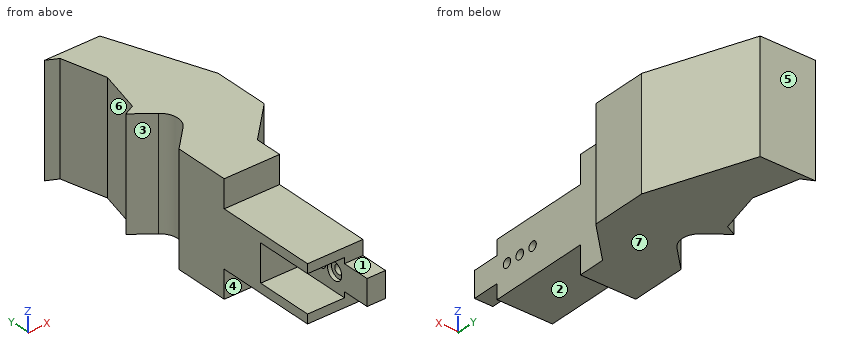
Autodesk Inventor part; units mm, degrees
ref_plane "Work Plane1" through (0, 0, -15) normal (0, 0, 1) x (1, 0, 0)
ref_plane "YZ Plane" through (0, 0, 0) normal (1, 0, 0) x (0, 1, 0)
ref_plane "XZ Plane" through (0, 0, 0) normal (0, 1, 0) x (-1, 0, 0)
sketch "Sketch1" plane through (0, 0, 0) normal (0, 0, 1) x (1, 0, 0)
  line L0 (0, 0) -> (25, 0)
  line L1 (25, 0) -> (25, 40)
  line L2 (25, 40) -> (0, 40)
  line L3 (0, 40) -> (0, 0)
  dimension "d1" = 25
  dimension "d2" = 40
  dimension "d3" = 25
extrude "Extrusion1" add sketch "Sketch1" against normal blind 30
sketch "Sketch2" plane through (25, 0, 0) normal (1, 0, 0) x (0, 0, -1)
  line L0 (0, 0) -> (30, 0)
  circle A0 centre (15, 6.56) radius 2.46
extrude "Extrusion2" cut sketch "Sketch2" against normal blind 30
sketch "Sketch3" plane through (0, 0, 0) normal (-1, 0, 0) x (0, 0, 1)
  line L0 (0, 0) -> (-30, 0)
  line L1 (-25.05, 0) -> (-4.95, 0)
  line L2 (-4.95, 0) -> (-4.95, 33.12)
  line L3 (-4.95, 33.12) -> (-25.05, 33.12)
  line L4 (-25.05, 33.12) -> (-25.05, 0)
  dimension "d11" = 20.1
extrude "Extrusion3" cut sketch "Sketch3" against normal blind 20
sketch "Sketch4" plane through (0, 0, 0) normal (0, -1, 0) x (1, 0, 0)
  line L0 (20, -4.95) -> (20, -25.05)
  line L1 (20, -15) -> (25, -15)
  line L2 (25, 0) -> (25, -30)
  line L3 (20, -8.025) -> (25, -8.025)
  line L4 (25, -8.025) -> (25, -21.975)
  line L5 (25, -21.975) -> (20, -21.975)
  line L6 (20, -21.975) -> (20, -8.025)
  line L7 (20, -8.025) -> (25, -21.975) construction
  line L8 (25, -8.025) -> (20, -21.975) construction
  line L9 (25, -12.54) -> (25, -17.46)
  point P0 (0, 0)
  point P1 (22.5, -15)
  dimension "d14" = 13.95
extrude "Extrusion4" add sketch "Sketch4" along normal blind 15
sketch "Sketch5" plane through (20, 0, 0) normal (-1, 0, 0) x (0, 0, 1)
  circle A0 centre (-15, 6.56) radius 2.46
  circle A1 centre (-15, 6.56) radius 4.7025
  circle A2 centre (-15, 6.56) radius 2.46
  circle A3 centre (-15, 6.56) radius 2.46
  point P0 (0, 0)
  dimension "d17" = 9.405
extrude "Extrusion5" cut sketch "Sketch5" against normal blind 2.1
sketch "Sketch6" plane through (25, 0, 0) normal (1, 0, 0) x (0, 0, -1)
  circle A0 centre (15, 6.56) radius 4.7025
  line L0 (15, 6.56) -> (15, 23.56)
  circle A1 centre (15, 23.56) radius 2.46
  point P0 (0, 0)
  dimension "d20" = 17
  dimension "d21" = 4.92
extrude "Extrusion6" cut sketch "Sketch6" against normal blind 10 contours A1
sketch "Sketch7" plane through (20, 0, 0) normal (-1, 0, 0) x (0, 0, 1)
  circle A0 centre (-15, 23.56) radius 2.46
  circle A1 centre (-15, 23.56) radius 4.7025
  point P0 (0, 0)
  dimension "d24" = 9.405
extrude "Extrusion7" cut sketch "Sketch7" against normal blind 2.1
sketch "Sketch9" plane through (25, 0, 0) normal (1, 0, 0) x (0, 0, -1)
  circle A0 centre (15, 6.56) radius 2.46
  circle A1 centre (15, 6.56) radius 2.46
  circle A2 centre (15, 23.56) radius 2.46
  circle A3 centre (15, 23.56) radius 2.46
  line L0 (30, 40) -> (30, 0)
  line L1 (30, 0) -> (30, 40)
  line L2 (30, 40) -> (0, 40)
  line L3 (0, 40) -> (0, 0)
  line L4 (0, 0) -> (8.025, 0)
  line L5 (21.975, 0) -> (21.975, -15)
  line L6 (21.975, -15) -> (8.025, -15)
  line L7 (8.025, -15) -> (8.025, 0)
  line L8 (0, 0) -> (8.025, 0)
  line L9 (21.975, 0) -> (30, 0)
extrude "Extrusion8" add sketch "Sketch9" along normal blind 5
sketch "Sketch10" plane through (0, 40, 0) normal (0, 1, 0) x (1, 0, 0)
  line L0 (0, 30) -> (30, 30)
  line L1 (30, 0) -> (0, 0)
  line L2 (0, 30) -> (30, 30)
  line L3 (30, 30) -> (30, 0)
  line L4 (30, 0) -> (0, 0)
  line L5 (0, 0) -> (0, 30)
extrude "Extrusion9" add sketch "Sketch10" along normal blind 30
sketch "Sketch12" plane through (30, 0, 0) normal (1, 0, 0) x (0, 0, -1)
  circle A0 centre (15, 6.56) radius 2.46
  line L0 (15, 6.56) -> (15, 15.06)
  circle A1 centre (15, 15.06) radius 2.525
  point P0 (0, 0)
  dimension "d31" = 8.5
  dimension "d33" = 5.05
extrude "Extrusion10" cut sketch "Sketch12" against normal blind 30 contours A1
sketch "Sketch15" plane through (0, 0, -25.05) normal (-1, 0, 0) x (0, 0, 1)
  line L0 (0, 33.12) -> (20.1, 33.12)
  line L1 (20.1, 33.12) -> (20.1, 0)
  line L2 (0, 33.12) -> (20.1, 33.12)
  line L3 (20.1, 33.12) -> (20.1, 31.1)
  line L4 (20.1, 31.1) -> (0, 31.1)
  line L5 (0, 31.1) -> (0, 33.12)
  point P0 (25.05, 0)
  dimension "d57" = 2.02
extrude "Extrusion13" add sketch "Sketch15" against normal blind 20
sketch "Sketch17" plane through (0, 0, 0) normal (0, 0, 1) x (1, 0, 0)
  line L0 (0, 70) -> (30, 70)
  line L1 (30, 70) -> (50.0622, 90.0622)
  line L2 (30, 70) -> (80, 70) construction
  line L3 (11.9522, 97.2454) -> (0, 85.2932)
  line L4 (0, 70) -> (0, 85.2932)
  line L5 (0, 70) -> (0, 0)
  line L6 (0, 70) -> (30, 70)
  line L7 (10.923, 112.2849) -> (0, 120.567)
  line L8 (50.0622, 105.3553) -> (50.0622, 120.567)
  line L9 (50.0622, 105.3553) -> (50.0622, 90.0622)
  arc A0 (11.9522, 97.2454) -> (10.923, 112.2849) centre (4.8811, 104.3165) ccw
  line L10 (0, 174.567) -> (30, 174.567)
  line L11 (30, 174.567) -> (50.0622, 120.567)
  line L12 (6, 171.567) -> (0, 174.567)
  line L13 (6, 123.567) -> (0, 120.567)
  line L14 (6, 123.567) -> (12, 147.567)
  line L15 (6, 171.567) -> (12, 147.567)
  dimension "d61" = 45
  dimension "d62" = 32.0271
  dimension "d72" = 10
extrude "Extrusion14" add sketch "Sketch17" against normal blind 30
sketch "Sketch24" plane through (0, 0, 0) normal (0, 0, 1) x (1, 0, 0)
  line L0 (30, 70) -> (50.0622, 90.0622)
  line L1 (30, 70) -> (50.0622, 90.0622)
  line L2 (50.0622, 90.0622) -> (50.0622, 120.567)
  line L3 (50.0622, 90.0622) -> (50.0622, 120.567)
  line L4 (30, 174.567) -> (50.0622, 120.567)
  line L5 (50.0622, 120.567) -> (30, 174.567)
  line L6 (30, 174.567) -> (0, 174.567)
  line L7 (30, 174.567) -> (0, 174.567)
  line L8 (0, 174.567) -> (6, 171.567)
  line L9 (0, 174.567) -> (6, 171.567)
  line L10 (12, 147.567) -> (6, 171.567)
  line L11 (6, 171.567) -> (12, 147.567)
  line L12 (12, 147.567) -> (6, 123.567)
  line L13 (12, 147.567) -> (6, 123.567)
  line L14 (6, 123.567) -> (0, 120.567)
  line L15 (6, 123.567) -> (0, 120.567)
  line L16 (0, 120.567) -> (10.923, 112.2849)
  line L17 (0, 120.567) -> (10.923, 112.2849)
  line L18 (0, 85.2932) -> (11.9522, 97.2454)
  line L19 (11.9522, 97.2454) -> (0, 85.2932)
  line L20 (0, 85.2932) -> (0, 55.2932)
  line L21 (0, 0) -> (0, 85.2932)
  line L22 (0, 55.2932) -> (30, 55.2932)
  line L23 (30, 0) -> (30, 70)
  line L24 (30, 55.2932) -> (30, 70)
  arc A0 (11.9522, 97.2454) -> (10.923, 112.2849) centre (4.8811, 104.3165) ccw
  dimension "d106" = 30
extrude "Extrusion15" add sketch "Sketch24" along normal blind 15
ref_plane "Work Plane1" through (0, 0, -15) normal (0, 0, 1) x (1, 0, 0)
mirror "Mirror1" about plane through (0, 0, -15) normal (0, 0, 1) of "Extrusion15"
properties part number "rec_c_48mm_x_60mm"
Input: part model. Units: mm. Frame: model coordinates. Face numbers are marked on the shaded views. A direction names the side the tool comes from. Coordinates: 2 decimals unless noted, no trailing zeros. Write each loop counter-clockwise with the first axis right and the second up, starting at its lowest first coordinate (ties: lowest second). Pieces come first, ordered by that corner, then holes. Notation, with made-up numbers: M -40,-6.5 L -29,-6.5 A33 ccw -29,32.5 Z; hole C -2.5,70 d7. An arc over 180 degrees is marked long. Use one line per item in the form item = value.
Q1. Section D-D (x = 9). Return loops of the section in (y, z), plus the area to 3 significant figures.
Answer below:
outline = M 0,-30 L 55.29,-30 L 55.29,-45 L 94.29,-45 L 94.29,15 L 55.29,15 L 55.29,0 L 0,0 L 0,-4.95 L 31.1,-4.95 L 31.1,-25.05 L 0,-25.05 Z; M 113.74,-45 L 135.57,-45 L 135.57,15 L 113.74,15 Z; M 159.57,-45 L 174.57,-45 L 174.57,15 L 159.57,15 Z
area = 5,580 mm²
Q2. Draft query along Y for the marked faces 4, 5, 6 and 7. Return one class per face: released by +Y, released by -Y, zero draft, split by the parting line, or undercut.
Answer below:
face_4 = released by -Y
face_5 = released by +Y
face_6 = undercut
face_7 = zero draft
Q3. Set-up query: the marked faces 1, 2 and 3. Return all of +Z, -Z, +X, -X, +Y, -Y with unobstructed straight access to the full face (end or side cutting, diameter ignored); none if empty.
Answer below:
face_1 = +Z, +X, -X, -Y
face_2 = -Z, +X, -X, -Y
face_3 = +Z, -Z, -X
Q4. Section B-B (x = 24.5). Return loops of the section in (y, z) (3 decimals), plus the area to 3 significant figures.
Answer below:
outline = M -15,-21.975 L 0,-21.975 L 0,-30 L 55.293,-30 L 55.293,-45 L 174.567,-45 L 174.567,15 L 55.293,15 L 55.293,0 L 0,0 L 0,-8.025 L -15,-8.025 Z; hole C 6.56,-15 d4.92; hole C 15.06,-15 d5.05; hole C 23.56,-15 d4.92
area = 8,970 mm²
Q5. Section A-A (y = 23.56). Return loops of the section in (x, z), plus the area to 3 significant figures.
Answer below:
outline = M 0,-30 L 30,-30 L 30,-17.46 L 22.1,-17.46 L 22.1,-19.7 L 20,-19.7 L 20,-25.05 L 0,-25.05 Z; M 0,-4.95 L 20,-4.95 L 20,-10.3 L 22.1,-10.3 L 22.1,-12.54 L 30,-12.54 L 30,0 L 0,0 Z
area = 439 mm²
Q6. Material intervals for probe 1 along Y at (x, z) = (27, -15) (3 decimals); probe 2 along Y at (x, z) = (21.65, -15) (1 decimal); probe 3 along X at (y, z) = (58, 4.5), sorted ascending. Write a range as from..to.
Answer below:
probe_1 = -15..4.1, 9.02..12.535, 17.585..21.1, 26.02..174.567
probe_2 = -15..1.9, 11.3..12.5, 17.6..18.9, 28.3..174.6
probe_3 = 0..30
Q7. First-contact query: pin 1 (8 mm diameter, centred on y = 23.56, z = -15, fed in from -X); pin 2 (16 mm diameter, centred on x = 7, y = 11, fed in from +Z); pin 3 (6 mm diameter, centred on y = 6, z = -13, fed in from -X). Flat tips, straight axial feed; report the tip coordinate or a pass-through.
Answer below:
pin_1 = 22.1
pin_2 = 0
pin_3 = 20
Q8. Section C-C (z = -2). Return loops of the section in (x, y), plus the area to 3 significant figures.
Answer below:
outline = M 0,0 L 30,0 L 30,70 L 50.06,90.06 L 50.06,120.57 L 30,174.57 L 0,174.57 L 6,171.57 L 12,147.57 L 6,123.57 L 0,120.57 L 10.92,112.28 A10 cw 11.95,97.25 L 0,85.29 Z
area = 5,820 mm²
